from build123d import *

# Parameters (mm, degrees)
EXTRUDE_1_DEPTH     = 20
SKETCH_2_W          = 5
SKETCH_2_H          = 10
CUT_EXTRUDE_1_DEPTH = 81.099407002


with BuildPart() as part:
    # Эскиз1 → Бобышка-Вытянуть1 (new body)
    with BuildSketch(Plane(origin=(0, 0, 0), x_dir=(1, 0, 0), z_dir=(0, 1, 0))):
        Polygon((0, 0), (10.099407002, 0), (10.099407002, 5), (20.099407002, 5), (20.099407002, 0), (30.099407002, 0), (30.099407002, 5), (40.099407002, 5), (40.099407002, 0), (50.099407002, 0), (50.099407002, 5), (60.099407002, 5), (60.099407002, 0), (70.099407002, 0), (70.099407002, 5), (80.099407002, 5), (80.099407002, 10), (0, 10), align=None)
    extrude(amount=EXTRUDE_1_DEPTH)

    # Эскиз2 → Вырез-Вытянуть1 (cut, through all)
    with BuildSketch(Plane.ZY):
        with Locations((-2.5, 15)):
            Rectangle(SKETCH_2_W, SKETCH_2_H)
    extrude(amount=-CUT_EXTRUDE_1_DEPTH, mode=Mode.SUBTRACT)


solid = part.part
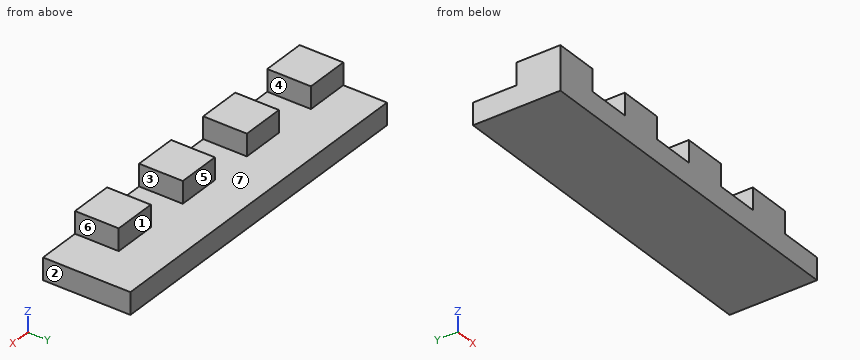
Source: CAD feature listing. Evaluate the final solid. Frame: model axes, mm. Face numbers are marked on the shaded views. A direction names the side the tool comes from. Round coordinates to 2 decimals unless told otherwise and drop trailing zeros. Loops run counter-clockwise (first coordinate to the right, second up) from the corner with the lowest first, then second, coordinate; pieces in that order, holes last.
Q1. First-contact query: P1, Ø6, axis at x = 26.5, y = 14.5, coming from the +Z side; P2, Ø4, axis at y = 7.5, z = -1.5, coming from the +X side; P3, Ø2.5, axis at x = 67, z = -3.5, coming from the +Y side. Flat tips, straight axial feed; report the tip coordinate or a pass-through.
Q2. Mould query, pull axis X, two halves, no side actions, for the marked faces 4, 5, 6 and 7. Classes: pulls with the +X half, pulls with the -X half, needs draft (parallel to the pull), parting line crosses it, or undercut.
Q3. Access query for the marked faces 1, 2 and 3. Directions: +Z, -Z, +X, -X, +Y, -Y. A direction counts if a zero-diameter tool reaches every point of the face in a straight line with its end or side. Return the directions, or none.
Q4. Section B-B, the plane y = 7.5. Return loops of the section in (x, z).
Q5. Ray query, line 1 (X direction, y = 1.25, z = -3.25); line 2 (Z direction, x = 16.5, y = 14.5); line 3 (Y direction, x = 28, z = -4.5). Return the intervals inside material, ascending.
Q6. Section C-C, the plane x = 42.5. Return loops of the section in (y, z), plus the area to 3 significant figures.
Q7. Section D-D, the plane y = 16. Return loops of the section in (x, z), plus the area to 3 significant figures.
Q8. Section A-A, the plane z = -0.75. Return loops of the section in (x, y), plus the area to 3 significant figures.
Solutions:
1. P1: stops at z = -5
1. P2: stops at x = 70.1
1. P3: stops at y = 10
2. face 4: undercut
2. face 5: needs draft
2. face 6: pulls with the +X half
2. face 7: undercut
3. face 1: +Z, +X, -X, +Y
3. face 2: +Z, -Z, +X, +Y, -Y
3. face 3: +Z, +Y, -Y
4. outline: (0, -10) - (80.1, -10) - (80.1, -5) - (70.1, -5) - (70.1, 0) - (60.1, 0) - (60.1, -5) - (50.1, -5) - (50.1, 0) - (40.1, 0) - (40.1, -5) - (30.1, -5) - (30.1, 0) - (20.1, 0) - (20.1, -5) - (10.1, -5) - (10.1, 0) - (0, 0) - close
5. line 1: x = 0 to 10.1, 20.1 to 30.1, 40.1 to 50.1, 60.1 to 70.1
5. line 2: z = -10 to -5
5. line 3: y = 0 to 10
6. outline: (0, -10) - (20, -10) - (20, -5) - (10, -5) - (10, 0) - (0, 0) - close
6. area: 150 mm2
7. outline: (0, -10) - (80.1, -10) - (80.1, -5) - (0, -5) - close
7. area: 400 mm2
8. outline: (0, 0) - (10.1, 0) - (10.1, 10) - (0, 10) - close; (20.1, 0) - (30.1, 0) - (30.1, 10) - (20.1, 10) - close; (40.1, 0) - (50.1, 0) - (50.1, 10) - (40.1, 10) - close; (60.1, 0) - (70.1, 0) - (70.1, 10) - (60.1, 10) - close
8. area: 401 mm2
